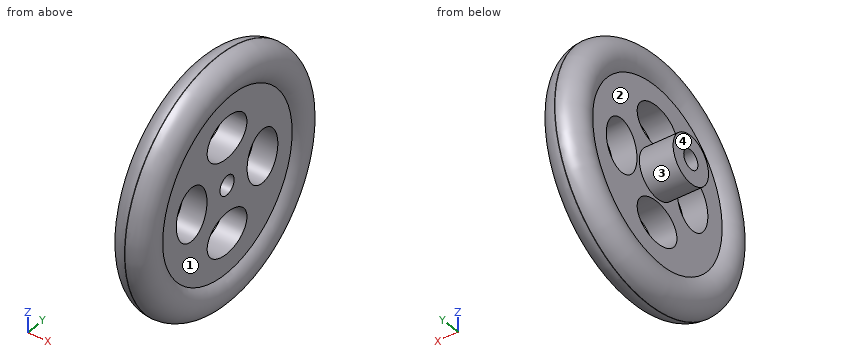
Autodesk Inventor part; units mm, degrees
ref_plane "YZ Plane" through (0, 0, 0) normal (1, 0, 0) x (0, 1, 0)
ref_plane "XZ Plane" through (0, 0, 0) normal (0, 1, 0) x (-1, 0, 0)
ref_plane "XY Plane" through (0, 0, 0) normal (0, 0, 1) x (1, 0, 0)
sketch "Skizze1" plane through (0, 0, 0) normal (0, 0, 1) x (1, 0, 0)
  line L0 (0, 0) -> (5, 0)
  line L1 (5, 0) -> (5, 21.5)
  line L2 (5, 21.5) -> (0, 21.5)
  line L3 (0, 21.5) -> (0, 0)
  circle A0 centre (2.5, 21.5) radius 4
  line L4 (0, 0) -> (-7, 0)
  line L5 (-7, 0) -> (-7, 5)
  line L6 (-7, 5) -> (0, 5)
  line L7 (0, 5) -> (0, 0)
  line L8 (2.45, 25.5) -> (2.55, 25.5)
  line L9 (2.5, 21.5) -> (2.5, 25.5) construction
  line L10 (2.45, 25.5) -> (2.45, 25.4997)
  line L11 (2.55, 25.5) -> (2.55, 25.4997)
  dimension "d0" = 8
  dimension "d1" = 21.5
  dimension "d2" = 5
  dimension "d3" = 7
  dimension "d4" = 5
  dimension "d9" = 0.1
revolve "Umdrehung1" add sketch "Skizze1" angle 360 about axis through (0, 0, 0) along (1, 0, 0)
sketch "Skizze2" plane through (-7, 0, 0) normal (-1, 0, 0) x (0, 0, 1)
  circle A0 centre (0, 0) radius 2
  dimension "d6" = 4
extrude "Extrusion1" cut sketch "Skizze2" against normal up to next
sketch "Skizze3" plane through (5, 0, 0) normal (1, 0, 0) x (0, 0, -1)
  line L0 (0, 0) -> (-10, 0) construction
  ellipse E0 centre (-10, 0) end of major axis (-10, 5.6146) minor radius 4.3356
  ellipse E1 centre (0, -10) end of major axis (-5.6146, -10) minor radius 4.3356
  ellipse E2 centre (10, 0) end of major axis (10, -5.6146) minor radius 4.3356
  ellipse E3 centre (0, 10) end of major axis (5.6146, 10) minor radius 4.3356
  dimension "d10" = 10
  dimension "d13" = 360
extrude "Extrusion2" cut sketch "Skizze3" against normal up to next
properties part number "Fake Rad" material "Aluminium 6061"
Verification items for the finished model (mm, model axes). Face numbers are marked on the shaded views. A direction names the side the tool comes from. Coordinates: 2 decimals unless noted, no trailing zeros. One line per item, written item: value. Start each with the question number.
Item 1: Access from +Z, -Z, +X, -X, +Y, -Y to the whole of each face (thin tool, end or side, straight path). Record for the marked faces 1 and 2.
Item 2: Thickness scan on probe 1 along X at (y, z) = (16.5, 4); probe 2 along X at (y, z) = (3, 0); probe 3 along Z at (x, y) = (0.25, -11.5). Record the ranges inside material, lowest first.
Item 3: Depth check by flat-ended pin: P1, Ø4, axis at x = 0, y = 16, coming from the -Z side; P2, Ø1, axis at x = -3.5, z = -10.5, coming from the +Y side; P3, Ø8, axis at x = 1.5, y = -4, coming from the -Z side; P4, Ø6.5, axis at y = 0, z = 0, coming from the +X side. Enter the tip coordinate at first touch or a pass-through.
Item 4: Sectioned sample at A-A on y = 0. Give the number of separate pieces and of enclosed holes in the cut face, then the cut area to 3 significant figures.
Item 5: Mould release check, pull along Z, two halves, no side actions. Record for the marked faces 3 and 4: pulls with the +Z half, pulls with the -Z half, needs draft (parallel to the pull), parting line crosses it, or undercut.
Calculated:
1. face 1: +X
1. face 2: -X
2. probe 1: 0 to 5
2. probe 2: -7 to 5
2. probe 3: -21.98 to -5.27, 5.27 to 21.98
3. P1: z = -20.79
3. P2: through
3. P3: z = -25.5
3. P4: x = 5
4. separate pieces: 4
4. enclosed holes: 0
4. area: 214 mm^2
5. face 3: undercut
5. face 4: needs draft
